Input: part model. Units: mm. Frame: model coordinates. Face numbers are marked on the shaded views. Give positions to 0.01 mm unless a question says otherwise; leave off trailing zeros. Order: outer loops, then holes, each group sorted by start corner. A loop starts at its lowest first (then second) coordinate and runs counter-clockwise, first axis right, second up.
```python
from build123d import *

# Parameters (mm, degrees)
CUERPO_DEPTH                  = 31
CROQUIS_HUECO_PCB_W           = 90.5
CROQUIS_HUECO_PCB_H           = 52.5
HUECO_PCB_DEPTH               = 29
CROQUIS_APOYOS_W              = 5
CROQUIS_APOYOS_H              = 5
APOYOS_PCB_DEPTH              = 4
CROQUIS_ALIVIOS_R             = 1
ALIVIOS_ESQUINAS_DEPTH        = 8.1
SALIDAS_USB_Y_PANEL_DEPTH     = 64.777935056
VENTILAS_LATERALES_DEPTH      = 64.777935056
VENTILAS_LATERALES_DEPTH_BACK = 64.777935056
REJILLA_PISO_DEPTH            = 2
CHAFLAN_BASE_SIZE             = 0.6


with BuildPart() as part:
    # Croquis_contorno → Cuerpo (new body)
    with BuildSketch(Plane(origin=(0, 0, 0), x_dir=(1, 0, 0), z_dir=(0, 1, 0))):
        with BuildLine():
            Line((-43.75, -28.75), (43.75, -28.75))
            ThreePointArc((43.75, -28.75), (46.578427125, -27.578427125), (47.75, -24.75))
            Line((47.75, -24.75), (47.75, 24.75))
            ThreePointArc((47.75, 24.75), (46.578427125, 27.578427125), (43.75, 28.75))
            Line((43.75, 28.75), (-43.75, 28.75))
            ThreePointArc((-43.75, 28.75), (-46.578427125, 27.578427125), (-47.75, 24.75))
            Line((-47.75, 24.75), (-47.75, -24.75))
            ThreePointArc((-47.75, -24.75), (-46.578427125, -27.578427125), (-43.75, -28.75))
        make_face()
    extrude(amount=CUERPO_DEPTH)

    # Croquis_hueco_PCB → Hueco_PCB (cut)
    with BuildSketch(Plane(origin=(0, 31, 0), x_dir=(1, 0, 0), z_dir=(0, 1, 0))):
        Rectangle(CROQUIS_HUECO_PCB_W, CROQUIS_HUECO_PCB_H)
    extrude(amount=-HUECO_PCB_DEPTH, mode=Mode.SUBTRACT)

    # Croquis_apoyos → Apoyos_PCB (add)
    with BuildSketch(Plane(origin=(0, 2, 0), x_dir=(1, 0, 0), z_dir=(0, 1, 0))):
        with Locations((-42.75, -23.75)):
            Rectangle(CROQUIS_APOYOS_W, CROQUIS_APOYOS_H)
        with Locations((-42.75, 23.75)):
            Rectangle(CROQUIS_APOYOS_W, CROQUIS_APOYOS_H)
        with Locations((42.75, -23.75)):
            Rectangle(CROQUIS_APOYOS_W, CROQUIS_APOYOS_H)
        with Locations((42.75, 23.75)):
            Rectangle(CROQUIS_APOYOS_W, CROQUIS_APOYOS_H)
    extrude(amount=APOYOS_PCB_DEPTH)

    # Croquis_alivios → Alivios_esquinas (cut)
    with BuildSketch(Plane(origin=(0, 2, 0), x_dir=(1, 0, 0), z_dir=(0, 1, 0))):
        with Locations(Location((-45.25, -26.25, 0), (0, 0, 90))):
            Circle(CROQUIS_ALIVIOS_R)
        with Locations(Location((-45.25, 26.25, 0), (0, 0, 270))):
            Circle(CROQUIS_ALIVIOS_R)
        with Locations(Location((45.25, -26.25, 0), (0, 0, 90))):
            Circle(CROQUIS_ALIVIOS_R)
        with Locations(Location((45.25, 26.25, 0), (0, 0, 270))):
            Circle(CROQUIS_ALIVIOS_R)
    extrude(amount=ALIVIOS_ESQUINAS_DEPTH, mode=Mode.SUBTRACT)

    # Croquis_salidas → Salidas_USB_y_panel (cut, through all)
    with BuildSketch(Plane.XY):
        with BuildLine():
            Line((6.8, 23.1), (11.8, 23.1))
            ThreePointArc((11.8, 23.1), (15.8, 19.1), (11.8, 15.1))
            Line((11.8, 15.1), (6.8, 15.1))
            ThreePointArc((6.8, 15.1), (2.8, 19.1), (6.8, 23.1))
        make_face()
        with BuildLine():
            Line((-15.96, 15.6), (-10.96, 15.6))
            ThreePointArc((-10.96, 15.6), (-7.46, 12.1), (-10.96, 8.6))
            Line((-10.96, 8.6), (-15.96, 8.6))
            ThreePointArc((-15.96, 8.6), (-19.46, 12.1), (-15.96, 15.6))
        make_face()
    extrude(amount=-SALIDAS_USB_Y_PANEL_DEPTH, mode=Mode.SUBTRACT)

    # Croquis_ventilas → Ventilas_laterales (cut, two sides: drawn at the far end of the back side and taken through both)
    with BuildSketch(Plane(origin=(0, 0, 0), x_dir=(0, 0, -1), z_dir=(1, 0, 0)).offset(-VENTILAS_LATERALES_DEPTH_BACK)):
        with BuildLine():
            Line((-20.859650045, 13.003805922), (-9.545941546, 24.317514421))
            ThreePointArc((-9.545941546, 24.317514421), (-7.424621202, 24.317514421), (-7.424621202, 22.196194078))
            Line((-7.424621202, 22.196194078), (-18.738329701, 10.882485579))
            ThreePointArc((-18.738329701, 10.882485579), (-20.859650045, 10.882485579), (-20.859650045, 13.003805922))
        make_face()
        with BuildLine():
            Line((-13.788582233, 13.003805922), (-2.474873734, 24.317514421))
            ThreePointArc((-2.474873734, 24.317514421), (-0.353553391, 24.317514421), (-0.353553391, 22.196194078))
            Line((-0.353553391, 22.196194078), (-11.66726189, 10.882485579))
            ThreePointArc((-11.66726189, 10.882485579), (-13.788582233, 10.882485579), (-13.788582233, 13.003805922))
        make_face()
        with BuildLine():
            Line((-6.717514421, 13.003805922), (4.596194078, 24.317514421))
            ThreePointArc((4.596194078, 24.317514421), (6.717514421, 24.317514421), (6.717514421, 22.196194078))
            Line((6.717514421, 22.196194078), (-4.596194078, 10.882485579))
            ThreePointArc((-4.596194078, 10.882485579), (-6.717514421, 10.882485579), (-6.717514421, 13.003805922))
        make_face()
        with BuildLine():
            Line((0.353553391, 13.003805922), (11.66726189, 24.317514421))
            ThreePointArc((11.66726189, 24.317514421), (13.788582233, 24.317514421), (13.788582233, 22.196194078))
            Line((13.788582233, 22.196194078), (2.474873734, 10.882485579))
            ThreePointArc((2.474873734, 10.882485579), (0.353553391, 10.882485579), (0.353553391, 13.003805922))
        make_face()
        with BuildLine():
            Line((7.424621202, 13.003805922), (18.738329701, 24.317514421))
            ThreePointArc((18.738329701, 24.317514421), (20.859650045, 24.317514421), (20.859650045, 22.196194078))
            Line((20.859650045, 22.196194078), (9.545941546, 10.882485579))
            ThreePointArc((9.545941546, 10.882485579), (7.424621202, 10.882485579), (7.424621202, 13.003805922))
        make_face()
    extrude(amount=VENTILAS_LATERALES_DEPTH + VENTILAS_LATERALES_DEPTH_BACK, mode=Mode.SUBTRACT)

    # Croquis_rejilla_piso → Rejilla_piso (cut)
    with BuildSketch(Plane(origin=(0, 0, 0), x_dir=(1, 0, 0), z_dir=(0, 1, 0))):
        with BuildLine():
            Line((-36.769552622, -13.435028843), (-7.778174593, 15.556349186))
            ThreePointArc((-7.778174593, 15.556349186), (-5.656854249, 15.556349186), (-5.656854249, 13.435028843))
            Line((-5.656854249, 13.435028843), (-34.648232278, -15.556349186))
            ThreePointArc((-34.648232278, -15.556349186), (-36.769552622, -15.556349186), (-36.769552622, -13.435028843))
        make_face()
        with BuildLine():
            Line((-29.69848481, -13.435028843), (-1.060660172, 15.202795796))
            ThreePointArc((-1.060660172, 15.202795796), (1.060660172, 15.202795796), (1.060660172, 13.081475452))
            Line((1.060660172, 13.081475452), (-27.577164466, -15.556349186))
            ThreePointArc((-27.577164466, -15.556349186), (-29.69848481, -15.556349186), (-29.69848481, -13.435028843))
        make_face()
        with BuildLine():
            Line((-22.273863607, -13.435028843), (6.363961031, 15.202795796))
            ThreePointArc((6.363961031, 15.202795796), (8.485281374, 15.202795796), (8.485281374, 13.081475452))
            Line((8.485281374, 13.081475452), (-20.152543264, -15.556349186))
            ThreePointArc((-20.152543264, -15.556349186), (-22.273863607, -15.556349186), (-22.273863607, -13.435028843))
        make_face()
        with BuildLine():
            Line((-15.379572491, -13.435028843), (13.258252147, 15.202795796))
            ThreePointArc((13.258252147, 15.202795796), (15.379572491, 15.202795796), (15.379572491, 13.081475452))
            Line((15.379572491, 13.081475452), (-13.258252147, -15.556349186))
            ThreePointArc((-13.258252147, -15.556349186), (-15.379572491, -15.556349186), (-15.379572491, -13.435028843))
        make_face()
        with BuildLine():
            Line((-7.954951288, -13.435028843), (20.68287335, 15.202795796))
            ThreePointArc((20.68287335, 15.202795796), (22.804193693, 15.202795796), (22.804193693, 13.081475452))
            Line((22.804193693, 13.081475452), (-5.833630945, -15.556349186))
            ThreePointArc((-5.833630945, -15.556349186), (-7.954951288, -15.556349186), (-7.954951288, -13.435028843))
        make_face()
        with BuildLine():
            Line((-1.060660172, -13.435028843), (27.577164466, 15.202795796))
            ThreePointArc((27.577164466, 15.202795796), (29.69848481, 15.202795796), (29.69848481, 13.081475452))
            Line((29.69848481, 13.081475452), (1.060660172, -15.556349186))
            ThreePointArc((1.060660172, -15.556349186), (-1.060660172, -15.556349186), (-1.060660172, -13.435028843))
        make_face()
        with BuildLine():
            Line((5.303300859, -13.435028843), (34.471455583, 15.733125881))
            ThreePointArc((34.471455583, 15.733125881), (36.592775926, 15.733125881), (36.592775926, 13.611805538))
            Line((36.592775926, 13.611805538), (7.424621202, -15.556349186))
            ThreePointArc((7.424621202, -15.556349186), (5.303300859, -15.556349186), (5.303300859, -13.435028843))
        make_face()
    extrude(amount=REJILLA_PISO_DEPTH, mode=Mode.SUBTRACT)

    # Chaflan_base
    chaflan_base_edges = [part.edges().sort_by_distance(p)[0] for p in [
        (47.75, 0, 0),
        (46.578427125, 0, 27.578427125),
        (0, 0, 28.75),
        (-46.578427125, 0, 27.578427125),
        (-47.75, 0, 0),
        (-46.578427125, 0, -27.578427125),
        (0, 0, -28.75),
        (46.578427125, 0, -27.578427125),
    ]]
    chamfer(chaflan_base_edges, length=CHAFLAN_BASE_SIZE)


solid = part.part
```
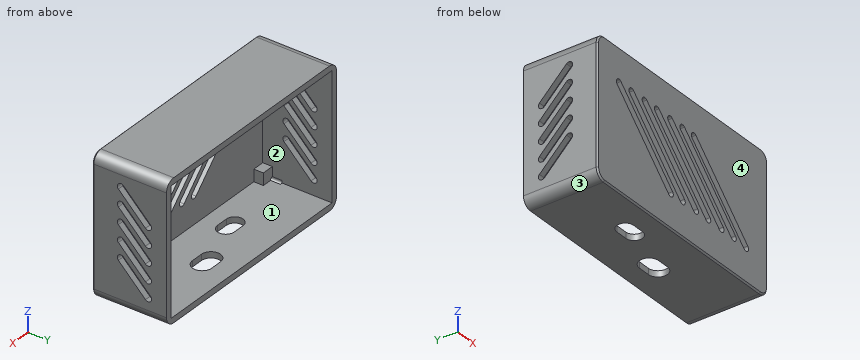
1) Line query: probe 1 along Z at (x, y) = (8.5, 6); probe 2 along X at (y, z) = (7, -19); probe 3 along Z at (x, y) = (12.5, 15.5). Output: solid intervals per line, ascending.
2) Cut plane C-C (x = -25.5). Return the cut outline in (y, z), then the cut area to 3 significant figures.
3) Cut plane B-B (y = 27.5). Return the cut outline in (x, z), then the cut area to 3 significant figures.
4) First-contact query: P1, Ø4, axis at x = -41.5, z = 24, coming from the +Y side. Flat tip, straight axial feed; report the tip coordinate or a pass-through.
5) Cut plane D-D (x = 32.5). Return the cut outline in (y, z), then the cut area to 3 significant figures.
6) Pull-direction query (X, two-part tool) for the marked faces 1, 2, 3 and 4; classes: pulls with the +X half, pulls with the -X half, needs draft (parallel to the pull), parting line crosses it, or undercut.
7) Cut plane A-A (y = 3.5). Return the cut outline in (x, z), then the cut area to 3 significant figures.
Geometry says:
1. probe 1: z = -28.75 to -26.25, 26.25 to 28.75
1. probe 2: x = -47.75 to -45.25, 45.25 to 47.75
1. probe 3: z = 26.25 to 28.75
2. outline: (0, -28.15) - (0.6, -28.75) - (31, -28.75) - (31, -26.25) - (2, -26.25) - (2, 2.17) - (0, 2.17) - close; (0, 6.41) - (2, 6.41) - (2, 9.24) - (0, 9.24) - close; (0, 13.48) - (2, 13.48) - (2, 26.25) - (31, 26.25) - (31, 28.75) - (0.6, 28.75) - (0, 28.15) - close
2. area: 243 mm2
3. outline: (-47.75, -24.75) arc R4 ccw to (-43.75, -28.75) - (43.75, -28.75) arc R4 ccw to (47.75, -24.75) - (47.75, 24.75) arc R4 ccw to (43.75, 28.75) - (-43.75, 28.75) arc R4 ccw to (-47.75, 24.75) - close; hole (-45.25, -26.25) - (45.25, -26.25) - (45.25, 26.25) - (-45.25, 26.25) - close
3. area: 726 mm2
4. P1: stops at y = 6
5. outline: (0, -28.15) - (0.6, -28.75) - (31, -28.75) - (31, -26.25) - (2, -26.25) - (2, -13.76) - (0, -13.76) - close; (0, -9.52) - (2, -9.52) - (2, 26.25) - (31, 26.25) - (31, 28.75) - (0.6, 28.75) - (0, 28.15) - close
5. area: 251 mm2
6. face 1: undercut
6. face 2: undercut
6. face 3: pulls with the -X half
6. face 4: needs draft
7. outline: (-47.75, -24.75) arc R4 ccw to (-43.75, -28.75) - (43.75, -28.75) arc R4 ccw to (47.75, -24.75) - (47.75, 24.75) arc R4 ccw to (43.75, 28.75) - (-43.75, 28.75) arc R4 ccw to (-47.75, 24.75) - close; hole circle Ø2 at (-45.25, -26.25); hole circle Ø2 at (-45.25, 26.25); hole (-45.25, -21.25) - (-40.25, -21.25) - (-40.25, -26.25) - (40.25, -26.25) - (40.25, -21.25) - (45.25, -21.25) - (45.25, 21.25) - (40.25, 21.25) - (40.25, 26.25) - (-40.25, 26.25) - (-40.25, 21.25) - (-45.25, 21.25) - close; hole circle Ø2 at (45.25, -26.25); hole circle Ø2 at (45.25, 26.25)
7. area: 814 mm2
